Build history of the part. All positions in model axes, mm. Face numbers are marked on the shaded views. A direction names the side the tool comes from. Coordinates: 2 decimals unless noted, no trailing zeros. Order: outer loops, then holes, each group sorted by start corner. A loop starts at its lowest first (then second) coordinate and runs counter-clockwise, first axis right, second up. Notation, with made-up numbers: (17, -39.5) - (44, -39.5) arc R11 ccw to (44, -23.5) - close; hole circle Ø5 at (84.25, 65.25). An arc over 180 degrees is marked (long way). Write each question's results on one line, items separated by ' | '.
from build123d import *

# Parameters (mm, degrees)
BOSS_EXTRU_1_DEPTH      = 11
BOSS_EXTRU_1_DEPTH_BACK = 11
ESQUISSE1_R             = 1.5
BOSS_EXTRU_3_DEPTH      = 3
BOSS_EXTRU_3_DEPTH_BACK = 25
BOSS_EXTRU_4_DEPTH      = 3
BOSS_EXTRU_5_DEPTH      = 3
ESQUISSE5_W             = 5
ESQUISSE5_H             = 2
ENL_V_MAT_EXTRU_1_DEPTH = 39
ESQUISSE6_W             = 5
ESQUISSE6_H             = 1.5
BOSS_EXTRU_6_DEPTH      = 28
BOSS_EXTRU_7_DEPTH      = 20
BOSS_EXTRU_7_DEPTH_BACK = 48


with BuildPart() as part:
    # Esquisse1 → Boss.-Extru.1 (new, two sides: drawn at the far end of the back side and taken through both)
    with BuildSketch(Plane(origin=(0, 0, 0), x_dir=(1, 0, 0), z_dir=(0, 1, 0)).offset(-BOSS_EXTRU_1_DEPTH_BACK)):
        with Locations(Location((0, 0, 0), (0, 0, 270))):
            Circle(ESQUISSE1_R)
    extrude(amount=BOSS_EXTRU_1_DEPTH + BOSS_EXTRU_1_DEPTH_BACK)



with BuildPart() as body_2:
    # Esquisse2 → Boss.-Extru.3 (new, two sides: drawn at the far end of the back side and taken through both)
    with BuildSketch(Plane.XZ.offset(11).offset(-BOSS_EXTRU_3_DEPTH_BACK)):
        Polygon((2.061683226, 10.308952687), (-3.759613912, 22.279872949), (-33.759613912, 22.279872949), (-33.759613912, 12.279872949), (-28.759613912, 12.279872949), (-28.759613912, 10.279872949), (-23.759613912, 10.279872949), (-23.759613912, 12.279872949), (-10.635382522, 12.279872949), (-8.075859571, 6.021220419), (2.061683226, 5.904476344), align=None)
    extrude(amount=BOSS_EXTRU_3_DEPTH + BOSS_EXTRU_3_DEPTH_BACK)


with BuildPart() as part_1:
    add(part.part)

    add(body_2.part)  # Boss.-Extru.4 merges body 2
    # Esquisse3 → Boss.-Extru.4 (add)
    with BuildSketch(Plane.XZ.offset(11)):
        Polygon((0, -1.5), (-6.831858839, -1.5), (-8.075859571, 6.021220419), (2.061683226, 5.904476344), (2.061683226, -1.5), align=None)
    extrude(amount=BOSS_EXTRU_4_DEPTH)

    # Esquisse4 → Boss.-Extru.5 (add)
    with BuildSketch(Plane(origin=(0, 11, 0), x_dir=(1, 0, 0), z_dir=(0, 1, 0))):
        Polygon((2.061683226, 1.5), (-6.831858839, 1.5), (-8.075859571, -6.021220419), (2.061683226, -5.904476344), align=None)
    extrude(amount=BOSS_EXTRU_5_DEPTH)

    # Esquisse5 → Enlèv. mat.-Extru.1 (cut)
    with BuildSketch(Plane(origin=(0, 14, 0), x_dir=(1, 0, 0), z_dir=(0, 1, 0))):
        with Locations((-26.259613912, -11.279872949)):
            Rectangle(ESQUISSE5_W, ESQUISSE5_H)
    extrude(amount=-ENL_V_MAT_EXTRU_1_DEPTH, mode=Mode.SUBTRACT)

    # Esquisse6 → Boss.-Extru.6 (add)
    with BuildSketch(Plane(origin=(0, 14, 0), x_dir=(1, 0, 0), z_dir=(0, 1, 0))):
        with Locations((-31.259613912, -11.529872949)):
            Rectangle(ESQUISSE6_W, ESQUISSE6_H)
    extrude(amount=-BOSS_EXTRU_6_DEPTH)

    # Esquisse7 → Boss.-Extru.7 (add, two sides: drawn at the far end of the back side and taken through both)
    with BuildSketch(Plane.XZ.offset(14).offset(-BOSS_EXTRU_7_DEPTH_BACK)):
        Polygon((2.061683226, 10.308952687), (-8.075859571, 6.021220419), (-10.635382522, 12.279872949), (-28.759613912, 12.279872949), (-28.759613912, 10.779872949), (-33.759613912, 10.779872949), (-33.759613912, 22.279872949), (-3.759613912, 22.279872949), align=None)
    extrude(amount=BOSS_EXTRU_7_DEPTH + BOSS_EXTRU_7_DEPTH_BACK)


solid = part_1.part
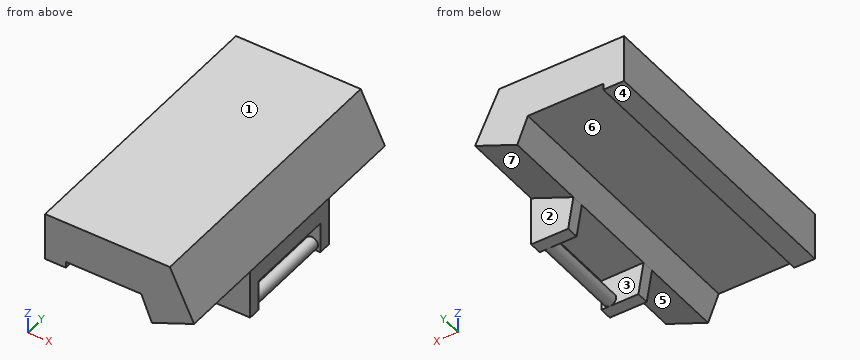
1. Tool access for the marked faces 4, 5, 6 and 7: list every direction of +Z, -Z, +X, -X, +Y, -Y with a clear straight run to the whole face (end or side of a thin tool).
Solved:
face 4: -Z, -X, +Y, -Y | face 5: -Z, +X, -Y | face 6: -Z, +Y, -Y | face 7: -Z, +X, +Y
2. Band-saw the part on D-D on x = -28. Give the cut face in (y, z), then the cut area to 3 significant figures.
Solved:
outline: (-34, 12.28) - (34, 12.28) - (34, 22.28) - (-34, 22.28) - close | area: 680 mm2
3. Two-plate mould, pull along Z, no slides. Class the marked faces 1, 2 and 3: +Z half, -Z half, draft (parallel to the pull), parting line (faces both ways), or undercut.
Solved:
face 1: +Z half | face 2: draft | face 3: undercut
4. Band-saw the part on A-A on y = -8.5. Give the cut face in (x, z), then the cut area to 3 significant figures.
Solved:
outline: (-33.76, 10.78) - (-28.76, 10.78) - (-28.76, 12.28) - (-10.64, 12.28) - (-8.08, 6.02) - (2.06, 5.9) - (2.06, 10.31) - (-3.76, 22.28) - (-33.76, 22.28) - close; circle Ø3 at (0, 0) | area: 410 mm2
5. Drop flat-ended pins along their axis: pin 1 Ø8 at (x, z) = (-3, 1.5) entering from -Y; pin 2 Ø3 at (x, y) = (-27, -2.5) entering from -Z; pin 3 Ø2.5 at (x, z) = (-3.5, 2.5) entering from +Y; pin 4 Ø4 at (y, z) = (-24, 3) entering from -X. Give the stop position or say it passes through.
Solved:
pin 1: stops at y = -14 | pin 2: stops at z = 12.28 | pin 3: stops at y = 14 | pin 4: passes through
6. Band-saw the part on B-B on y = -21. Give the cut face in (x, z), then the cut area to 3 significant figures.
Solved:
outline: (-33.76, 10.78) - (-28.76, 10.78) - (-28.76, 12.28) - (-10.64, 12.28) - (-8.08, 6.02) - (2.06, 10.31) - (-3.76, 22.28) - (-33.76, 22.28) - close | area: 381 mm2
7. Band-saw the part on C-C on z = 9. Give the cut face in (x, y), then the cut area to 3 significant figures.
Solved:
outline: (-9.29, -34) - (-1.03, -34) - (-1.03, -14) - (2.06, -14) - (2.06, 14) - (-1.03, 14) - (-1.03, 34) - (-9.29, 34) - close | area: 648 mm2
8. Probe line 1 (Z direction, x = -22, y = -23.5); line 2 (Y direction, x = -4, z = 6.5); line 3 (Z direction, x = -1, y = 6.5) (3 decimals). List the from-to ranges inside material, lowest first.
Solved:
line 1: z = 12.28 to 22.28 | line 2: y = -14 to 14 | line 3: z = -1.118 to 1.118, 5.94 to 16.605
